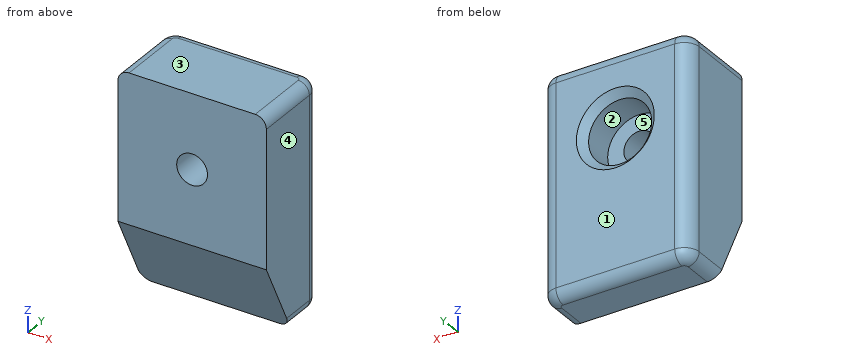
```python
from build123d import *

# Parameters (mm, degrees)
SKETCH1_W           = 40
SKETCH1_H           = 60
SKETCH1_R           = 4.15
BOSS_EXTRUDE1_DEPTH = 11
SKETCH2_R           = 8.5
CUT_EXTRUDE1_DEPTH  = 10
FILLET1_R           = 4
CHAMFER1_SIZE       = 2
CHAMFER2_SIZE       = 20
CHAMFER2_SIZE2      = 10
FILLET2_R           = 3


with BuildPart() as part:
    # Sketch1 → Boss-Extrude1 (new body, symmetric)
    with BuildSketch(Plane(origin=(0, 0, 0), x_dir=(1, 0, 0), z_dir=(0, 1, 0))):
        with Locations((0, 0.089127558)):
            Rectangle(SKETCH1_W, SKETCH1_H)
        with Locations((0, -9.910872442)):
            Circle(SKETCH1_R, mode=Mode.SUBTRACT)
    extrude(amount=BOSS_EXTRUDE1_DEPTH, both=True)

    # Sketch2 → Cut-Extrude1 (cut)
    with BuildSketch(Plane(origin=(0, 11, 0), x_dir=(1, 0, 0), z_dir=(0, 1, 0))):
        with Locations((0, -9.910872442)):
            Circle(SKETCH2_R)
    extrude(amount=-CUT_EXTRUDE1_DEPTH, mode=Mode.SUBTRACT)

    # Fillet1
    fillet1_edges = [part.edges().sort_by_distance(p)[0] for p in [
        (-20, 11, -0.089127558),
        (20, 11, -0.089127558),
    ]]
    fillet(fillet1_edges, radius=FILLET1_R)

    # Chamfer1
    chamfer1_edges = [part.edges().sort_by_distance(p)[0] for p in [
        (-8.5, 11, 9.910872442),
    ]]
    chamfer(chamfer1_edges, length=CHAMFER1_SIZE)

    # Chamfer2
    chamfer2_edges = [part.edges().sort_by_distance(p)[0] for p in [
        (0, -11, -30.089127558),
    ]]
    chamfer2_side = [part.faces().sort_by_distance(p)[0] for p in [
        (0, -11, -0.319769187),
    ]]
    chamfer(chamfer2_edges, length=CHAMFER2_SIZE, length2=CHAMFER2_SIZE2, reference=chamfer2_side[0])

    # Fillet2
    fillet2_edges = [part.edges().sort_by_distance(p)[0] for p in [
        (0, 11, -30.089127558),
        (0, 11, 29.910872442),
        (20, -2, 29.910872442),
        (-20, -2, 29.910872442),
        (18.828427125, 9.828427125, 29.910872442),
        (-18.828427125, 9.828427125, 29.910872442),
        (-20, 3, -30.089127558),
        (20, 3, -30.089127558),
        (18.828427125, 9.828427125, -30.089127558),
        (-18.828427125, 9.828427125, -30.089127558),
    ]]
    fillet(fillet2_edges, radius=FILLET2_R)


solid = part.part
```
Source: CAD feature listing. Evaluate the final solid. Frame: model axes, mm. Face numbers are marked on the shaded views. A direction names the side the tool comes from. Coordinates: 2 decimals unless noted, no trailing zeros. Loops run counter-clockwise (first coordinate to the right, second up) from the corner with the lowest first, then second, coordinate; pieces in that order, holes last. Notation, with made-up numbers: M 88,-8 L 144,-8 A14 ccw 144,10 Z; hole C 52,-36.5 d3. An arc over 180 degrees is marked long. Put each result on its own line as item: value. Start each with the question number.
1) Pull-direction query (X, two-part tool) for the marked faces 3, 4 and 5; classes: pulls with the +X half, pulls with the -X half, needs draft (parallel to the pull), parting line crosses it, or undercut.
2) Ray query, L1, parallel to Z at x = 0, y = 4; L2, parallel to X at y = 2.75, z = 10; L3, parallel to X at y = 9.25, z = 17. Return the intervals inside material, ascending. Write a range as from..to.
3) Reachability of the marked faces 1 and 2 from +Z, -Z, +X, -X, +Y, -Y: full face, straight path, thin tool, end or side. Return the list, or none.
4) Cut plane C-C on y = 2. Return the cut outline in (x, z).
5) Contact query for flat-ended pins moving along their axis: pin 1 Ø15.5 at (x, z) = (0, 9.91) entering from -Y; pin 2 Ø11 at (x, z) = (0, 9.91) entering from +Y. Output: stop coordinate, or through.
6) Cut plane D-D on z = -17. Return the cut outline in (x, y), then the cut area to 3 significant figures.
7) Cut plane A-A on x = 0. Return the cut outline in (y, z).
8) Cut plane B-B on x = 15. Return the cut outline in (y, z).
The answers:
1. face 3: needs draft
1. face 4: pulls with the +X half
1. face 5: undercut
2. L1: z = -30.09..1.41, 18.41..29.91
2. L2: x = -20..-8.5, 8.5..20
2. L3: x = -19.31..-5.13, 5.13..19.31
3. face 1: +Z, -Z, +X, -X, +Y
3. face 2: +Y
4. outline: M -20,-27.09 A3 ccw -17,-30.09 L 17,-30.09 A3 ccw 20,-27.09 L 20,26.91 A3 ccw 17,29.91 L -17,29.91 A3 ccw -20,26.91 Z; hole C 0,9.91 d17
5. pin 1: stops at y = -11
5. pin 2: stops at y = 1
6. outline: M -20,-7.54 L 20,-7.54 L 20,7 A4 ccw 16,11 L -16,11 A4 ccw -20,7 Z
6. area: 735 mm²
7. outline: M -11,-10.09 L -1,-30.09 L 8,-30.09 A3 ccw 11,-27.09 L 11,-0.59 L 9,1.41 L 1,1.41 L 1,5.76 L -11,5.76 Z; M -11,14.06 L 1,14.06 L 1,18.41 L 9,18.41 L 11,20.41 L 11,26.91 A3 ccw 8,29.91 L -11,29.91 Z
8. outline: M -11,-10.09 L -1,-30.09 L 8,-30.09 A3 ccw 11,-27.09 L 11,26.91 A3 ccw 8,29.91 L -11,29.91 Z
